```python
from build123d import *

# Parameters (mm, degrees)
F0_W     = 360
F0_H     = 19
F1_DEPTH = 5
F3_DEPTH = 25
F4_R     = 1


with BuildPart() as f1:
    # F0 (on Front) → F1 (new body)
    with BuildSketch(Plane.XZ):
        Rectangle(F0_W, F0_H)
    extrude(amount=F1_DEPTH)

    # F2 (on face) → F3 (cut)
    with BuildSketch(Plane.XZ.offset(5)):
        Polygon((-29.716518, 0), (-40, -9.5), (40, -9.5), (29.716518, 0), align=None)
    extrude(amount=-F3_DEPTH, mode=Mode.SUBTRACT)

    # F4
    f4_edges = [f1.edges().sort_by_distance(p)[0] for p in [
        (0, -5, 9.5),
        (0, 0, 9.5),
        (110, -5, -9.5),
        (-110, -5, -9.5),
        (0, -5, 0),
        (34.858259, -5, -4.75),
        (-34.858259, -5, -4.75),
        (110, 0, -9.5),
        (-110, 0, -9.5),
        (0, 0, 0),
        (-34.858259, 0, -4.75),
        (34.858259, 0, -4.75),
    ]]
    fillet(f4_edges, radius=F4_R)


solid = f1.part
```
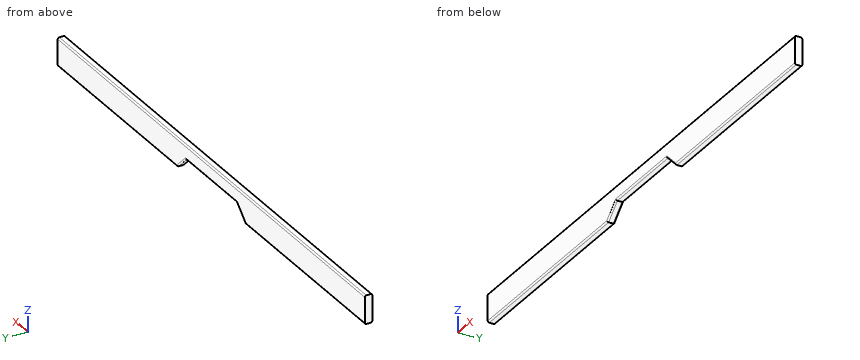
Could you check a few things on this model? Use its own coordinates, in mm. Round coordinates to 2 decimals unless told otherwise and drop trailing zeros. Loops run counter-clockwise (first coordinate to the right, second up) from the corner with the lowest first, then second, coordinate; pieces in that order, holes last. Notation, with made-up numbers: M 78,-28.5 L 85,-28.5 A24 ccw 85,-8.5 Z; hole C 47,-5.75 d6. An arc over 180 degrees is marked long. Put each result on its own line as item: value.
Q1. For pin 1 (0.9 mm diameter, centred on x = -0.5, y = -3, fed in from -Z), with a flat end and sliding along its axis, tell me the tip position at first contact or that it passes through.
Check result:
pin 1: z = 0
Q2. Imagine slicing it at B-B (x = -23.5). Write out the boundary of the cut face in (y, z).
Check result:
outline: M -5,1 A1 ccw -4,0 L -1,0 A1 ccw 0,1 L 0,8.5 A1 ccw -1,9.5 L -4,9.5 A1 ccw -5,8.5 Z
Q3. I need wall thicknesses on probe 1 along X at (y, z) = (-3, -2.25); probe 2 along Z at (x, y) = (1, -3.75); probe 3 along X at (y, z) = (-1.5, -3.5). Which ranges of each line are inside material? Lowest first, please.
Check result:
probe 1: -180 to -32.15, 32.15 to 180
probe 2: 0 to 9.5
probe 3: -180 to -33.51, 33.51 to 180
Q4. Imagine slicing it at A-A (y = -3.1). Write out the boundary of the cut face in (x, z).
Check result:
outline: M -180,-9.5 L -40,-9.5 L -29.72,0 L 29.72,0 L 40,-9.5 L 180,-9.5 L 180,9.5 L -180,9.5 Z
